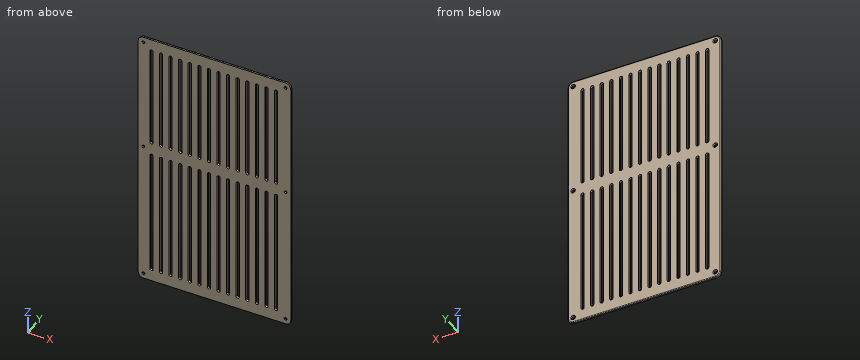
```python
from build123d import *

# Parameters (mm, degrees)
SKETCH1_R           = 1.75
BOSS_EXTRUDE1_DEPTH = 3
CHAMFER1_SIZE       = 1.1
CUT_EXTRUDE1_DEPTH  = 38
CUT_EXTRUDE2_DEPTH  = 10
FILLET1_R           = 1


with BuildPart() as part:
    # Sketch1 → Boss-Extrude1 (new body)
    with BuildSketch(Plane(origin=(0, 0, 0), x_dir=(1, 0, 0), z_dir=(0, 1, 0))):
        with BuildLine():
            Line((0, 7), (0, 315))
            ThreePointArc((0, 315), (2.050252532, 319.949747468), (7, 322))
            Line((7, 322), (185, 322))
            ThreePointArc((185, 322), (189.949747468, 319.949747468), (192, 315))
            Line((192, 315), (192, 7))
            ThreePointArc((192, 7), (189.949747468, 2.050252532), (185, 0))
            Line((185, 0), (7, 0))
            ThreePointArc((7, 0), (2.050252532, 2.050252532), (0, 7))
        make_face()
        with Locations(Location((7, 315, 0), (0, 0, 270))):
            Circle(SKETCH1_R, mode=Mode.SUBTRACT)
        with Locations(Location((185, 315, 0), (0, 0, 270))):
            Circle(SKETCH1_R, mode=Mode.SUBTRACT)
        with Locations(Location((185, 7, 0), (0, 0, 270))):
            Circle(SKETCH1_R, mode=Mode.SUBTRACT)
        with Locations(Location((7, 7, 0), (0, 0, 270))):
            Circle(SKETCH1_R, mode=Mode.SUBTRACT)
        with Locations(Location((7, 146, 0), (0, 0, 270))):
            Circle(SKETCH1_R, mode=Mode.SUBTRACT)
        with Locations(Location((185, 146, 0), (0, 0, 270))):
            Circle(SKETCH1_R, mode=Mode.SUBTRACT)
    extrude(amount=BOSS_EXTRUDE1_DEPTH)

    # Chamfer1
    chamfer1_edges = [part.edges().sort_by_distance(p)[0] for p in [
        (7, 3, -316.75),
        (185, 3, -316.75),
        (185, 3, -8.75),
        (7, 3, -8.75),
        (7, 3, -147.75),
        (185, 3, -147.75),
    ]]
    chamfer(chamfer1_edges, length=CHAMFER1_SIZE)

    # Sketch2 → Cut-Extrude1 (cut)
    with BuildSketch(Plane(origin=(0, 3, 0), x_dir=(1, 0, 0), z_dir=(0, 1, 0))):
        with BuildLine():
            Line((31.1, 306), (31.1, 155))
            ThreePointArc((31.1, 155), (29.1, 153), (27.1, 155))
            Line((27.1, 155), (27.1, 306))
            ThreePointArc((27.1, 306), (29.1, 308), (31.1, 306))
        make_face()
        with BuildLine():
            Line((31.1, 16), (31.1, 137.46))
            ThreePointArc((31.1, 137.46), (29.1, 139.46), (27.1, 137.46))
            Line((27.1, 137.46), (27.1, 16))
            ThreePointArc((27.1, 16), (29.1, 14), (31.1, 16))
        make_face()
        with BuildLine():
            Line((15.1, 306), (15.1, 155))
            ThreePointArc((15.1, 155), (17.1, 153), (19.1, 155))
            Line((19.1, 155), (19.1, 306))
            ThreePointArc((19.1, 306), (17.1, 308), (15.1, 306))
        make_face()
        with BuildLine():
            Line((43.1, 306), (43.1, 155))
            ThreePointArc((43.1, 155), (41.1, 153), (39.1, 155))
            Line((39.1, 155), (39.1, 306))
            ThreePointArc((39.1, 306), (41.1, 308), (43.1, 306))
        make_face()
        with BuildLine():
            Line((43.1, 16), (43.1, 137.46))
            ThreePointArc((43.1, 137.46), (41.1, 139.46), (39.1, 137.46))
            Line((39.1, 137.46), (39.1, 16))
            ThreePointArc((39.1, 16), (41.1, 14), (43.1, 16))
        make_face()
        with BuildLine():
            Line((15.1, 16), (15.1, 137.46))
            ThreePointArc((15.1, 137.46), (17.1, 139.46), (19.1, 137.46))
            Line((19.1, 137.46), (19.1, 16))
            ThreePointArc((19.1, 16), (17.1, 14), (15.1, 16))
        make_face()
        with BuildLine():
            Line((55.1, 306), (55.1, 155))
            ThreePointArc((55.1, 155), (53.1, 153), (51.1, 155))
            Line((51.1, 155), (51.1, 306))
            ThreePointArc((51.1, 306), (53.1, 308), (55.1, 306))
        make_face()
        with BuildLine():
            Line((55.1, 16), (55.1, 137.46))
            ThreePointArc((55.1, 137.46), (53.1, 139.46), (51.1, 137.46))
            Line((51.1, 137.46), (51.1, 16))
            ThreePointArc((51.1, 16), (53.1, 14), (55.1, 16))
        make_face()
        with BuildLine():
            Line((67.1, 306), (67.1, 155))
            ThreePointArc((67.1, 155), (65.1, 153), (63.1, 155))
            Line((63.1, 155), (63.1, 306))
            ThreePointArc((63.1, 306), (65.1, 308), (67.1, 306))
        make_face()
        with BuildLine():
            Line((67.1, 16), (67.1, 137.46))
            ThreePointArc((67.1, 137.46), (65.1, 139.46), (63.1, 137.46))
            Line((63.1, 137.46), (63.1, 16))
            ThreePointArc((63.1, 16), (65.1, 14), (67.1, 16))
        make_face()
        with BuildLine():
            Line((79.1, 306), (79.1, 155))
            ThreePointArc((79.1, 155), (77.1, 153), (75.1, 155))
            Line((75.1, 155), (75.1, 306))
            ThreePointArc((75.1, 306), (77.1, 308), (79.1, 306))
        make_face()
        with BuildLine():
            Line((79.1, 16), (79.1, 137.46))
            ThreePointArc((79.1, 137.46), (77.1, 139.46), (75.1, 137.46))
            Line((75.1, 137.46), (75.1, 16))
            ThreePointArc((75.1, 16), (77.1, 14), (79.1, 16))
        make_face()
        with BuildLine():
            Line((91.1, 306), (91.1, 155))
            ThreePointArc((91.1, 155), (89.1, 153), (87.1, 155))
            Line((87.1, 155), (87.1, 306))
            ThreePointArc((87.1, 306), (89.1, 308), (91.1, 306))
        make_face()
        with BuildLine():
            Line((91.1, 16), (91.1, 137.46))
            ThreePointArc((91.1, 137.46), (89.1, 139.46), (87.1, 137.46))
            Line((87.1, 137.46), (87.1, 16))
            ThreePointArc((87.1, 16), (89.1, 14), (91.1, 16))
        make_face()
        with BuildLine():
            Line((103.1, 306), (103.1, 155))
            ThreePointArc((103.1, 155), (101.1, 153), (99.1, 155))
            Line((99.1, 155), (99.1, 306))
            ThreePointArc((99.1, 306), (101.1, 308), (103.1, 306))
        make_face()
        with BuildLine():
            Line((103.1, 16), (103.1, 137.46))
            ThreePointArc((103.1, 137.46), (101.1, 139.46), (99.1, 137.46))
            Line((99.1, 137.46), (99.1, 16))
            ThreePointArc((99.1, 16), (101.1, 14), (103.1, 16))
        make_face()
        with BuildLine():
            Line((115.1, 306), (115.1, 155))
            ThreePointArc((115.1, 155), (113.1, 153), (111.1, 155))
            Line((111.1, 155), (111.1, 306))
            ThreePointArc((111.1, 306), (113.1, 308), (115.1, 306))
        make_face()
        with BuildLine():
            Line((115.1, 16), (115.1, 137.46))
            ThreePointArc((115.1, 137.46), (113.1, 139.46), (111.1, 137.46))
            Line((111.1, 137.46), (111.1, 16))
            ThreePointArc((111.1, 16), (113.1, 14), (115.1, 16))
        make_face()
        with BuildLine():
            Line((127.1, 306), (127.1, 155))
            ThreePointArc((127.1, 155), (125.1, 153), (123.1, 155))
            Line((123.1, 155), (123.1, 306))
            ThreePointArc((123.1, 306), (125.1, 308), (127.1, 306))
        make_face()
        with BuildLine():
            Line((127.1, 16), (127.1, 137.46))
            ThreePointArc((127.1, 137.46), (125.1, 139.46), (123.1, 137.46))
            Line((123.1, 137.46), (123.1, 16))
            ThreePointArc((123.1, 16), (125.1, 14), (127.1, 16))
        make_face()
        with BuildLine():
            Line((139.1, 306), (139.1, 155))
            ThreePointArc((139.1, 155), (137.1, 153), (135.1, 155))
            Line((135.1, 155), (135.1, 306))
            ThreePointArc((135.1, 306), (137.1, 308), (139.1, 306))
        make_face()
        with BuildLine():
            Line((139.1, 16), (139.1, 137.46))
            ThreePointArc((139.1, 137.46), (137.1, 139.46), (135.1, 137.46))
            Line((135.1, 137.46), (135.1, 16))
            ThreePointArc((135.1, 16), (137.1, 14), (139.1, 16))
        make_face()
        with BuildLine():
            Line((151.1, 306), (151.1, 155))
            ThreePointArc((151.1, 155), (149.1, 153), (147.1, 155))
            Line((147.1, 155), (147.1, 306))
            ThreePointArc((147.1, 306), (149.1, 308), (151.1, 306))
        make_face()
        with BuildLine():
            Line((151.1, 16), (151.1, 137.46))
            ThreePointArc((151.1, 137.46), (149.1, 139.46), (147.1, 137.46))
            Line((147.1, 137.46), (147.1, 16))
            ThreePointArc((147.1, 16), (149.1, 14), (151.1, 16))
        make_face()
        with BuildLine():
            Line((163.1, 306), (163.1, 155))
            ThreePointArc((163.1, 155), (161.1, 153), (159.1, 155))
            Line((159.1, 155), (159.1, 306))
            ThreePointArc((159.1, 306), (161.1, 308), (163.1, 306))
        make_face()
        with BuildLine():
            Line((163.1, 16), (163.1, 137.46))
            ThreePointArc((163.1, 137.46), (161.1, 139.46), (159.1, 137.46))
            Line((159.1, 137.46), (159.1, 16))
            ThreePointArc((159.1, 16), (161.1, 14), (163.1, 16))
        make_face()
        with BuildLine():
            Line((175.1, 306), (175.1, 155))
            ThreePointArc((175.1, 155), (173.1, 153), (171.1, 155))
            Line((171.1, 155), (171.1, 306))
            ThreePointArc((171.1, 306), (173.1, 308), (175.1, 306))
        make_face()
        with BuildLine():
            Line((175.1, 16), (175.1, 137.46))
            ThreePointArc((175.1, 137.46), (173.1, 139.46), (171.1, 137.46))
            Line((171.1, 137.46), (171.1, 16))
            ThreePointArc((171.1, 16), (173.1, 14), (175.1, 16))
        make_face()
    extrude(amount=-CUT_EXTRUDE1_DEPTH, mode=Mode.SUBTRACT)

    # Sketch3 → Cut-Extrude2 (cut)
    with BuildSketch(Plane.XZ):
        with BuildLine():
            Line((185, 0), (7, 0))
            ThreePointArc((7, 0), (2.050252532, -2.050252532), (0, -7))
            Line((0, -7), (0, -315))
            ThreePointArc((0, -315), (2.050252532, -319.949747468), (7, -322))
            Line((7, -322), (185, -322))
            ThreePointArc((185, -322), (189.949747468, -319.949747468), (192, -315))
            Line((192, -315), (192, -7))
            ThreePointArc((192, -7), (189.949747468, -2.050252532), (185, 0))
        make_face()
        with BuildLine():
            Line((185, -0.5), (7, -0.5))
            ThreePointArc((7, -0.5), (2.403805922, -2.403805922), (0.5, -7))
            Line((0.5, -7), (0.5, -315))
            ThreePointArc((0.5, -315), (2.403805922, -319.596194078), (7, -321.5))
            Line((7, -321.5), (185, -321.5))
            ThreePointArc((185, -321.5), (189.596194078, -319.596194078), (191.5, -315))
            Line((191.5, -315), (191.5, -7))
            ThreePointArc((191.5, -7), (189.596194078, -2.403805922), (185, -0.5))
        make_face(mode=Mode.SUBTRACT)
    extrude(amount=-CUT_EXTRUDE2_DEPTH, mode=Mode.SUBTRACT)

    # Fillet1
    fillet1_edges = [part.edges().sort_by_distance(p)[0] for p in [
        (189.596194078, 3, -2.403805922),
        (191.5, 3, -161),
        (189.596194078, 3, -319.596194078),
        (96, 3, -321.5),
        (2.403805922, 3, -319.596194078),
        (0.5, 3, -161),
        (2.403805922, 3, -2.403805922),
        (96, 3, -0.5),
    ]]
    fillet(fillet1_edges, radius=FILLET1_R)


solid = part.part
```
The listing builds one solid part. Answer for the finished solid, in the listing's coordinates (mm). Round coordinates to 2 decimals unless told otherwise and drop trailing zeros.
Q1. Section A-A, the plane y = 1 is taken. Count the separate pieces of the cut face and the enclosed holes in it, then the cut area to 3 significant figures.
Q2. Find the intervals of material crossed by line 1 (X direction, y = 1.2, z = -146); line 2 (Z direction, x = 185, y = 1.3); line 3 (Z direction, x = 140.5, y = 2.3), in increasing order.
Q3. Given pin 1 Ø1.5 at (x, z) = (31.5, -242.5) entering from -Y; pin 2 Ø3 at (x, z) = (185, -146) entering from +Y, each flat-ended and moving along its own axis, determine where each tip first touches the part or whether it passes through.
Completed:
1. separate pieces: 1
1. enclosed holes: 34
1. area: 45,600 mm2
2. line 1: x = 0.5 to 5.25, 8.75 to 183.25, 186.75 to 191.5
2. line 2: z = -321.5 to -316.75, -313.25 to -147.75, -144.25 to -8.75, -5.25 to -0.5
2. line 3: z = -321.45 to -0.55
3. pin 1: stops at y = 0
3. pin 2: passes through
